Part model, mm, in its own coordinate system. A direction names the side the tool comes from. Round coordinates to 2 decimals unless told otherwise and drop trailing zeros. Order: outer loops, then holes, each group sorted by start corner. A loop starts at its lowest first (then second) coordinate and runs counter-clockwise, first axis right, second up. Notation, with made-up numbers: (-1, 31.5) -> (12, 31.5) arc R13 ccw to (12, 39.5) -> close; hole circle Ø5 at (-16.75, -36). An arc over 180 degrees is marked (long way). Use CSV: the item, a comma, the result in double quotes.
```python
from build123d import *

# Parameters (mm, degrees)
SKETCH1_R           = 22.987
SKETCH1_R_2         = 1.905
BOSS_EXTRUDE1_DEPTH = 6.35


with BuildPart() as part:
    # Sketch1 → Boss-Extrude1 (new body)
    with BuildSketch(Plane(origin=(0, 0, 0), x_dir=(1, 0, 0), z_dir=(0, 1, 0))):
        Circle(SKETCH1_R)
        with Locations((0, 19.84375)):
            Circle(SKETCH1_R_2, mode=Mode.SUBTRACT)
        with Locations((17.185191606, 9.921875)):
            Circle(SKETCH1_R_2, mode=Mode.SUBTRACT)
        with Locations((17.185191606, -9.921875)):
            Circle(SKETCH1_R_2, mode=Mode.SUBTRACT)
        with Locations((0, -19.84375)):
            Circle(SKETCH1_R_2, mode=Mode.SUBTRACT)
        with Locations((-17.185191606, -9.921875)):
            Circle(SKETCH1_R_2, mode=Mode.SUBTRACT)
        with Locations((-17.185191606, 9.921875)):
            Circle(SKETCH1_R_2, mode=Mode.SUBTRACT)
        with BuildLine():
            Line((-7.065939428, -6.35), (7.065939428, -6.35))
            ThreePointArc((7.065939428, -6.35), (9.5, 0), (7.065939428, 6.35))
            Line((7.065939428, 6.35), (-7.065939428, 6.35))
            ThreePointArc((-7.065939428, 6.35), (-9.5, 0), (-7.065939428, -6.35))
        make_face(mode=Mode.SUBTRACT)
    extrude(amount=BOSS_EXTRUDE1_DEPTH)


solid = part.part
```
(1) Drop flat-ended pins along their axis: P1, Ø1.5, axis at x = -5.5, y = 5.5, coming from the +Z side; P2, Ø3, axis at y = 3, z = -2, coming from the -X side; P3, Ø3, axis at x = -2, y = 2.5, coming from the -Z side. Give the stop position or say it passes through.
Reply:
P1,"z = 22.49"
P2,"x = -22.98"
P3,"z = -22.98"
(2) Cut at C-C, the plane y = 2.75. Give the cut face in (x, z) (3 decimals), then the cut area to 3 significant figures.
Reply:
outline,"circle Ø45.974 at (0, 0); hole circle Ø3.81 at (-17.185, -9.922); hole circle Ø3.81 at (-17.185, 9.922); hole (-7.066, -6.35) -> (7.066, -6.35) arc R9.5 ccw to (7.066, 6.35) -> (-7.066, 6.35) arc R9.5 ccw to start; hole circle Ø3.81 at (0, -19.844); hole circle Ø3.81 at (0, 19.844); hole circle Ø3.81 at (17.185, -9.922); hole circle Ø3.81 at (17.185, 9.922)"
area,"1,370 mm2"
(3) Cut at A-A, the plane z = 0. Give the cut face in (x, y).
Reply:
outline,"(-22.99, 0) -> (-9.5, 0) -> (-9.5, 6.35) -> (-22.99, 6.35) -> close; (9.5, 0) -> (22.99, 0) -> (22.99, 6.35) -> (9.5, 6.35) -> close"
(4) Probe probe 1 along Z at (x, y) = (0, 4); probe 2 along X at (y, z) = (1, -9); probe 3 along Z at (x, y) = (0.5, 2.5). List the from-to ranges inside material, lowest first. Write a range as [from, to].
Reply:
probe 1,"[-22.99, -21.75], [-17.94, -6.35], [6.35, 17.94], [21.75, 22.99]"
probe 2,"[-21.15, -18.85], [-15.52, 15.52], [18.85, 21.15]"
probe 3,"[-22.98, -21.68], [-18.01, -6.35], [6.35, 18.01], [21.68, 22.98]"
(5) Pull direction Z, two halves, no side cores. Call faces 3 (the face through (12.36, 3.13, -19.38)), 4 (the face through (-15.37, 3.13, 9.35)), 5 (the face through (10, 6.35, 0)), 6 (the face through (-0.413, 3.131, 21.703)): released by +Z, released by -Z, zero draft, split by the parting line, or undercut.
Reply:
face 3,"split by the parting line"
face 4,"undercut"
face 5,"zero draft"
face 6,"undercut"
(6) Which spindle directions (+Z, -Z, +X, -X, +Y, -Y) get a long thin tool onto all of the face, cutting with end or side? Do faces 1 (the face through (-9.5, 3.1, -0.1)), 2 (the face through (10, 0, 0)). Say none if no direction does.
Reply:
face 1,"+Y, -Y"
face 2,"+Z, -Z, +X, -X, -Y"
(7) Cut at B-B, the plane x = 0. Give the cut face in (y, z), then the cut area to 3 significant figures.
Reply:
outline,"(0, -22.99) -> (6.35, -22.99) -> (6.35, -21.75) -> (0, -21.75) -> close; (0, -17.94) -> (6.35, -17.94) -> (6.35, -6.35) -> (0, -6.35) -> close; (0, 6.35) -> (6.35, 6.35) -> (6.35, 17.94) -> (0, 17.94) -> close; (0, 21.75) -> (6.35, 21.75) -> (6.35, 22.99) -> (0, 22.99) -> close"
area,"163 mm2"
(8) Cut at D-D, the plane z = 5.5. Give the cut face in (x, y).
Reply:
outline,"(-22.32, 0) -> (-7.75, 0) -> (-7.75, 6.35) -> (-22.32, 6.35) -> close; (7.75, 0) -> (22.32, 0) -> (22.32, 6.35) -> (7.75, 6.35) -> close"
